Answer from the drawing. Dimensions are ordinates in mm from the lowest x, y and z of the part. A direction names the side the tool comes from. Give positions to 0.01 mm unless a question says otherwise; leave off trailing zeros. Loops run counter-clockwise (first coordinate to the right, second up) from the corner with the lowest first, then second, coordinate; pieces in that order, holes last.
(1) Find section B-B, the plane z = 4.5. Write down the section's boundary in (x, y), then the cut area to 3 significant figures.
(2) Find section A-A, the plane y = 2.5. State how many separate pieces and enclosed holes the cut face has.
(3) Straight lines are drawn through the part: probe 1 along X at (y, z) = (0.9, 6); probe 2 along Z at (x, y) = (1.5, 3.5); probe 3 along Y at (x, z) = (4, 0.5). For each, find the intervals that lie inside material, in ascending order.
(4) Each of these flat-tipped pins is pushed along its axis until it touches: P1, Ø2, axis at x = 3, y = 3, coming from the +Z side; P2, Ø1, axis at y = 2.5, z = 4.5, coming from the +X side; P3, Ø2, axis at y = 3.5, z = 5, coming from the -X side. Where does it stop, or does it pass through?
(5) Determine the mould class of the marked faces 3, 4, 5 and 6 for opening direction Z: pulls with the +Z half, pulls with the -Z half, needs draft (parallel to the pull), parting line crosses it, or undercut.
(6) Find section D-D, the plane y = 4.25. Write down the section's boundary in (x, z), then the cut area to 3 significant figures.
(7) Which of the six approach directions +Z, -Z, +X, -X, +Y, -Y give full straight-line access (tool end or side, diameter ignored) to the marked faces 1 and 2?
(8) Find section C-C, the plane x = 4.5. Write down the section's boundary in (y, z).
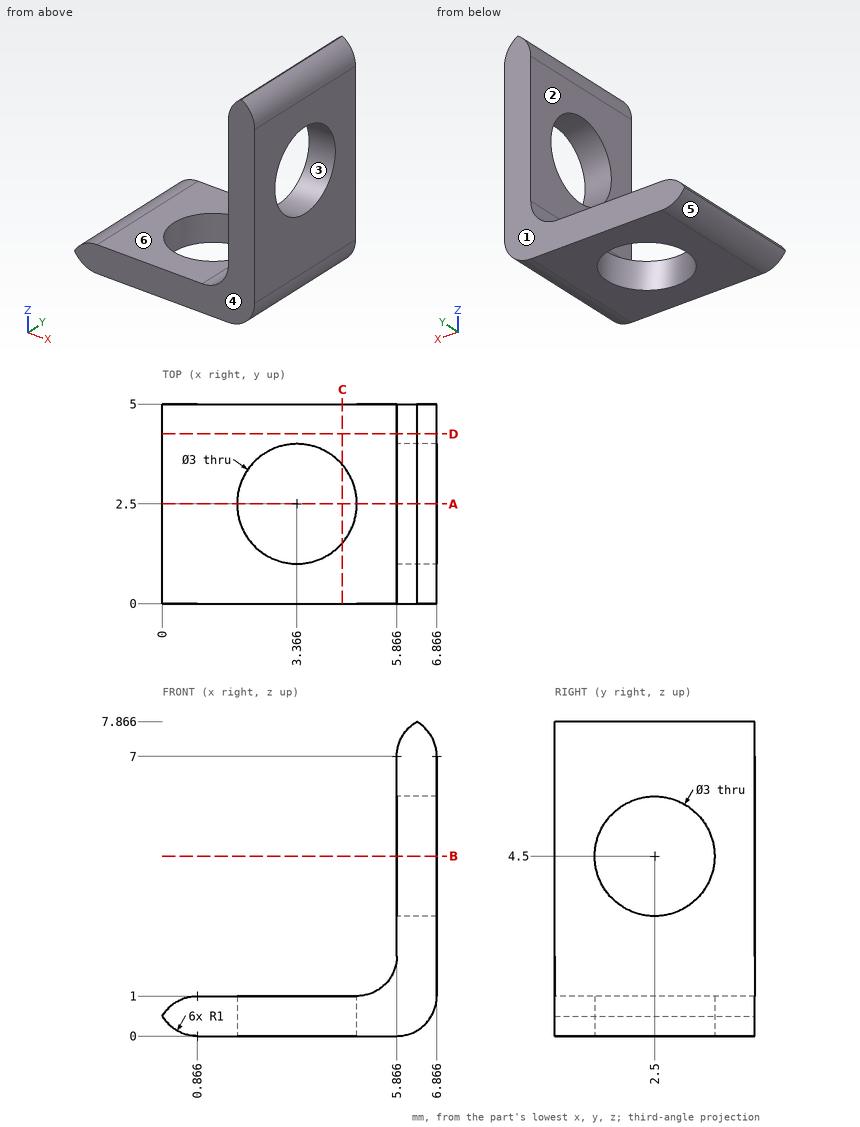
Entries:
1. outline: (5.87, 0) - (6.87, 0) - (6.87, 1) - (5.87, 1) - close; (5.87, 4) - (6.87, 4) - (6.87, 5) - (5.87, 5) - close
1. area: 2.00 mm2
2. separate pieces: 3
2. enclosed holes: 0
3. probe 1: x = 5.87 to 6.87
3. probe 2: z = 0 to 1
3. probe 3: y = 0 to 1.14, 3.86 to 5
4. P1: stops at z = 1
4. P2: passes through
4. P3: stops at x = 5.87
5. face 3: undercut
5. face 4: needs draft
5. face 5: pulls with the -Z half
5. face 6: pulls with the +Z half
6. outline: (0, 0.5) arc R1 ccw to (0.87, 0) - (5.87, 0) arc R1 ccw to (6.87, 1) - (6.87, 7) arc R1 ccw to (6.37, 7.87) arc R1 ccw to (5.87, 7) - (5.87, 2) arc R1 cw to (4.87, 1) - (0.87, 1) arc R1 ccw to start
6. area: 13.2 mm2
7. face 1: +Z, -Z, +X, -X, +Y
7. face 2: +Z, -X, +Y, -Y
8. outline: (0, 0) - (1.52, 0) - (1.52, 1) - (0, 1) - close; (3.48, 0) - (5, 0) - (5, 1) - (3.48, 1) - close
